Could you check a few things on this model? Use its own coordinates, in mm. A direction names the side the tool comes from. Give positions to 0.01 mm unless a question says otherwise; leave off trailing zeros. Order: outer loops, then holes, each group sorted by start corner. A loop starts at its lowest first (then second) coordinate and runs counter-clockwise, first axis right, second up.
(1) Will these pins go through, and if not, where does the flat tip stop? pin 1 (1 mm diameter, centred on y = 2, z = -1, fed in from +X); pin 2 (1.5 mm diameter, centred on x = -8, z = 0.5, fed in from -Y).
(2) On a 3-axis mill with a long thin cutter (end or side, diameter ignored), from which of +Z, -Z, +X, -X, +Y, -Y can I reach the whole of each face in a straight line? I mean faces 1 (the flat face through (9.503, 0, 0)), 2 (the cylindrical face through (8.02, -1.22, 0.27)). Say none if no direction works.
(3) Imagine slicing it at C-C, the plane x = -14.5. Write out the boundary of the cut face in (y, z), then the cut area to 3 significant figures.
(4) If I drill on probe 1 along X at (y, z) = (0.7, 1.6); probe 2 along X at (y, z) = (-1.35, -0.55); probe 3 along Z at (x, y) = (3.5, 1.45), over which ranges is the centre line in solid material (lowest first)?
(5) Imagine slicing it at D-D, the plane x = 3.5. Write out the boundary of the cut face in (y, z), then the cut area to 3 significant figures.
(6) Imagine slicing it at A-A, the plane y = 0. Write out the boundary of the cut face in (x, z), then the cut area to 3 significant figures.
from build123d import *

# Parameters (mm, degrees)
CHAMFER1_SIZE = 0.3


with BuildPart() as part:
    # Sketch2 → Revolve1 (revolve)
    with BuildSketch(Plane(origin=(0, 0, 0), x_dir=(1, 0, 0), z_dir=(0, 1, 0))):
        Polygon((-16.496503497, 2.5), (-11.496503497, 2.5), (-11.496503497, 1.6), (6.503496503, 1.6), (6.503496503, 1.25), (9.503496503, 1.25), (9.503496503, 0), (-16.496503497, 0), align=None)
    revolve(axis=Axis((-6.153846154, 0, 0), (1, 0, 0)))

    # Chamfer1
    chamfer1_edges = [part.edges().sort_by_distance(p)[0] for p in [
        (-16.496503497, 0, 2.5),
        (-11.496503497, 0, 2.5),
    ]]
    chamfer(chamfer1_edges, length=CHAMFER1_SIZE)


solid = part.part
Answer block:
1. pin 1: stops at x = -11.5
1. pin 2: stops at y = -1.6
2. face 1: +Z, -Z, +X, +Y, -Y
2. face 2: +X
3. outline: circle Ø5 at (0, 0)
3. area: 19.6 mm2
4. probe 1: x = -16.5 to -11.5
4. probe 2: x = -16.5 to 6.5
4. probe 3: z = -0.68 to 0.68
5. outline: circle Ø3.2 at (0, 0)
5. area: 8.04 mm2
6. outline: (-16.5, -2.2) - (-16.2, -2.5) - (-11.8, -2.5) - (-11.5, -2.2) - (-11.5, -1.6) - (6.5, -1.6) - (6.5, -1.25) - (9.5, -1.25) - (9.5, 1.25) - (6.5, 1.25) - (6.5, 1.6) - (-11.5, 1.6) - (-11.5, 2.2) - (-11.8, 2.5) - (-16.2, 2.5) - (-16.5, 2.2) - close
6. area: 89.9 mm2
